```python
from build123d import *

# Parameters (mm, degrees)
SKETCH1_W           = 25
SKETCH1_H           = 45
BOSS_EXTRUDE1_DEPTH = 12
M5_TAPPED_HOLE1_D   = 4.2
M5_TAPPED_HOLE2_D   = 4.2


with BuildPart() as part:
    # Sketch1 → Boss-Extrude1 (new body)
    with BuildSketch(Plane(origin=(0, 0, 0), x_dir=(1, 0, 0), z_dir=(0, 1, 0))):
        Rectangle(SKETCH1_W, SKETCH1_H)
    extrude(amount=BOSS_EXTRUDE1_DEPTH)

    # M5 Tapped Hole1 (through all)
    with Locations(Plane(origin=(0, 12, 0), x_dir=(1, 0, 0), z_dir=(0, 1, 0))):
        with Locations((7.5, 18), (-7.5, -18)):
            Hole(M5_TAPPED_HOLE1_D / 2)

    # M5 Tapped Hole2 (through all)
    with Locations(Plane(origin=(12.5, 0, 0), x_dir=(0, 0, -1), z_dir=(1, 0, 0))):
        with Locations((0, 6)):
            Hole(M5_TAPPED_HOLE2_D / 2)


solid = part.part
```
The model under review builds one solid part; all positions refer to its coordinate system, in mm. Coordinates: 2 decimals unless noted, no trailing zeros. Write each loop counter-clockwise with the first axis right and the second up, starting at its lowest first coordinate (ties: lowest second). Pieces come first, ordered by that corner, then holes.
1) We need section A-A on x = 7.5. State the section outline as (y, z) points.
2) The part is to be moulded in two halves that separate along X. For faces 1 (the face through (-7.227, 5.916, 15.918)), 2 (the face through (0, 6, 22.5)), 3 (the face through (12.5, 3, 0)), 4 (the face through (-12.5, 3, 0)), say which applies: pulls with the +X half, pulls with the -X half, needs draft (parallel to the pull), parting line crosses it, or undercut.
3) We need section D-D on y = 11. State the section outline as (x, z) points.
4) We need section B-B on y = 6. State the section outline as (x, z) points, then the cut area to 3 significant figures.
5) To check wall thickness, follow probe 1 along X at (y, z) = (4.5, -18); probe 2 along Z at (x, y) = (6.5, 7); probe 3 along Z at (x, y) = (-7.5, 9.25). State the ranges of each line that lie inside material, in increasing order.
6) We need section C-C on z = 0. State the section outline as (x, y) points.
Answer list:
1. outline: (0, -22.5) - (12, -22.5) - (12, -20.1) - (0, -20.1) - close; (0, -15.9) - (12, -15.9) - (12, 22.5) - (0, 22.5) - close; hole circle Ø4.2 at (6, 0)
2. face 1: undercut
2. face 2: needs draft
2. face 3: pulls with the +X half
2. face 4: pulls with the -X half
3. outline: (-12.5, -22.5) - (12.5, -22.5) - (12.5, 22.5) - (-12.5, 22.5) - close; hole circle Ø4.2 at (-7.5, 18); hole circle Ø4.2 at (7.5, -18)
4. outline: (-12.5, -22.5) - (12.5, -22.5) - (12.5, -2.1) - (-12.5, -2.1) - close; (-12.5, 2.1) - (12.5, 2.1) - (12.5, 22.5) - (-12.5, 22.5) - close; hole circle Ø4.2 at (-7.5, 18); hole circle Ø4.2 at (7.5, -18)
4. area: 992 mm2
5. probe 1: x = -12.5 to 5.4, 9.6 to 12.5
5. probe 2: z = -22.5 to -19.85, -16.15 to -1.85, 1.85 to 22.5
5. probe 3: z = -22.5 to 15.9, 20.1 to 22.5
6. outline: (-12.5, 0) - (12.5, 0) - (12.5, 3.9) - (-12.5, 3.9) - close; (-12.5, 8.1) - (12.5, 8.1) - (12.5, 12) - (-12.5, 12) - close
